Read the model definition and answer for the solid it produces. Units are mm, in the model's axes. Coordinates: 2 decimals unless noted, no trailing zeros. Write each loop counter-clockwise with the first axis right and the second up, starting at its lowest first coordinate (ties: lowest second). Pieces come first, ordered by that corner, then holes.
1) This flat-tipped pin is pushed along its axis until it touches: pin 1 Ø6 at (x, y) = (-3, 1) entering from -Z. Where does it stop, or does it pass through?
2) Find the intervals of material crossed by line 1 (X direction, y = -33.5, z = 1.5); line 2 (Y direction, x = -9, z = 0.3); line 3 (Y direction, x = -10.75, z = 1.6), in increasing order.
3) The part is cut by section A-A (z = 0.6). Determine the outline of the cut face in (x, y) (3 decimals), then the cut area to 3 significant figures.
4) The part is cut by section C-C (x = -7.5). Determine the outline of the cut face in (y, z), then the cut area to 3 significant figures.
5) The part is cut by section B-B (y = -24). Determine the outline of the cut face in (x, z).
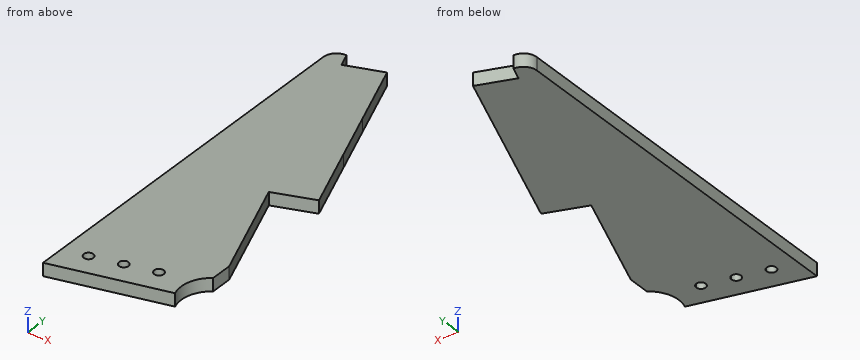
from build123d import *

# Parameters (mm, degrees)
F1_DEPTH = 1.7018


with BuildPart() as f1:
    # F0 (on Top) → F1 (new body)
    with BuildSketch(Plane.XY):
        with BuildLine():
            Line((-13.194016, 9.354334), (-13.856456, 11.104334))
            ThreePointArc((-13.856456, 11.104334), (-15.093893, 10.591771), (-15.606456, 9.354334))
            Line((-15.606456, 9.354334), (-15.606456, -36.036127))
            Line((-15.606456, -36.036127), (-15.606456, -39.141956))
            Line((-15.606456, -39.141956), (-1.117569, -35.25967))
            ThreePointArc((-1.117569, -35.25967), (-1.198453, -32.663077), (0.332721, -30.564424))
            Line((0.332721, -30.564424), (0.332721, -27.792238))
            Line((0.332721, -27.792238), (-4.811083, -14.203604))
            Line((-4.811083, -14.203604), (0.332721, -12.256482))
            Line((0.332721, -12.256482), (-2.853478, -3.839349))
            Line((-2.853478, -3.839349), (-5.331632, 2.707311))
            Line((-5.331632, 2.707311), (-8.510218, 11.104334))
            Line((-8.510218, 11.104334), (-8.570957, 11.104334))
            Line((-8.570957, 11.104334), (-13.194016, 9.354334))
        make_face()
        with BuildLine():
            ThreePointArc((-11.951597, -35.224279), (-12.495019, -35.843932), (-13.180301, -35.386041))
            ThreePointArc((-13.180301, -35.386041), (-12.738359, -34.620576), (-11.972894, -35.062517))
            ThreePointArc((-11.972894, -35.062517), (-11.956944, -35.1427), (-11.951597, -35.224279))
        make_face(mode=Mode.SUBTRACT)
        with BuildLine():
            ThreePointArc((-8.087894, -34.189003), (-8.631315, -34.808656), (-9.316598, -34.350765))
            ThreePointArc((-9.316598, -34.350765), (-8.874656, -33.585299), (-8.10919, -34.027241))
            ThreePointArc((-8.10919, -34.027241), (-8.093241, -34.107424), (-8.087894, -34.189003))
        make_face(mode=Mode.SUBTRACT)
        with BuildLine():
            ThreePointArc((-4.224191, -33.153727), (-4.767612, -33.77338), (-5.452894, -33.315489))
            ThreePointArc((-5.452894, -33.315489), (-4.93077, -32.534074), (-4.224191, -33.153727))
        make_face(mode=Mode.SUBTRACT)
    extrude(amount=F1_DEPTH)


solid = f1.part
Reported:
1. pin 1: stops at z = 0
2. line 1: x = -15.61 to -5.37, -4.33 to -1.36
2. line 2: y = -37.37 to -34.74, -33.63 to 10.94
2. line 3: y = -37.84 to 10.28
3. outline: (-15.606, -39.142) - (-1.118, -35.26) arc R4 cw to (0.333, -30.564) - (0.333, -27.792) - (-4.811, -14.204) - (0.333, -12.256) - (-2.853, -3.839) - (-8.51, 11.104) - (-8.571, 11.104) - (-13.194, 9.354) - (-13.856, 11.104) arc R1.75 ccw to (-15.606, 9.354) - close; hole (-11.973, -35.063) arc R0.625 ccw (long way) to (-11.952, -35.224) arc R0.625 ccw to start; hole (-8.109, -34.027) arc R0.625 ccw (long way) to (-8.088, -34.189) arc R0.625 ccw to start; hole circle Ø1.25 at (-4.849, -33.154)
3. area: 609 mm2
4. outline: (-36.97, 0) - (8.44, 0) - (8.44, 1.7) - (-36.97, 1.7) - close
4. area: 77.3 mm2
5. outline: (-15.61, 0) - (-1.1, 0) - (-1.1, 1.7) - (-15.61, 1.7) - close
